from build123d import *

# Parameters (mm, degrees)
SKETCH1_R                = 10.5
BOSS_EXTRUDE1_DEPTH      = 2
SKETCH1_2_R              = 10.5
BOSS_EXTRUDE2_DEPTH      = 2
SKETCH2_R                = 12.5
SKETCH2_R_2              = 10.5
BOSS_EXTRUDE3_DEPTH      = 3.015
BOSS_EXTRUDE3_DEPTH_BACK = 3.015


with BuildPart() as part:
    # Sketch1 → Boss-Extrude1 (new body)
    with BuildSketch(Plane(origin=(0, 0, 0), x_dir=(1, 0, 0), z_dir=(0, 1, 0))):
        Circle(SKETCH1_R)
    extrude(amount=BOSS_EXTRUDE1_DEPTH)

    # Sketch1_2 → Boss-Extrude2 (add)
    with BuildSketch(Plane(origin=(0, 0, 0), x_dir=(1, 0, 0), z_dir=(0, 1, 0))):
        Circle(SKETCH1_2_R)
    extrude(amount=-BOSS_EXTRUDE2_DEPTH)

    # Sketch2 → Boss-Extrude3 (add, two sides)
    with BuildSketch(Plane(origin=(0, 0, 0), x_dir=(1, 0, 0), z_dir=(0, 1, 0))) as boss_extrude3_sk:
        Circle(SKETCH2_R)
        Circle(SKETCH2_R_2, mode=Mode.SUBTRACT)
    extrude(amount=BOSS_EXTRUDE3_DEPTH)
    extrude(boss_extrude3_sk.sketch, amount=-BOSS_EXTRUDE3_DEPTH_BACK)


solid = part.part
Part model, mm, in its own coordinate system. A direction names the side the tool comes from. Coordinates: 2 decimals unless noted, no trailing zeros. Order: outer loops, then holes, each group sorted by start corner. A loop starts at its lowest first (then second) coordinate and runs counter-clockwise, first axis right, second up. Notation, with made-up numbers: M 12.5,25 L 69.5,25 A16 cw 69.5,35 Z; hole C 84.5,-30.75 d5. An arc over 180 degrees is marked long. One line per question, with ' | ' between items.
Q1. Slice it at B-B (x = 0). Give the cut face in (y, z) (3 decimals), and give its area (3 significant figures).
A:
outline: M -3.015,-12.5 L 3.015,-12.5 L 3.015,-10.5 L 2,-10.5 L 2,10.5 L 3.015,10.5 L 3.015,12.5 L -3.015,12.5 L -3.015,10.5 L -2,10.5 L -2,-10.5 L -3.015,-10.5 Z | area: 108 mm^2
Q2. Pin check, flat tips, straight feed: P1, Ø2, axis at x = 1, z = -8.5, coming from the -Y side; P2, Ø1.5, axis at x = -6.5, y = 2.5, coming from the +Z side; P3, Ø1, axis at y = -0.5, z = 3.5, coming from the -X side; P4, Ø3, axis at x = 1, y = -2, coming from the +Z side. Stop position of each tip, or through.
A:
P1: stops at y = -2 | P2: stops at z = 11.1 | P3: stops at x = -12.13 | P4: stops at z = 12.5
Q3. Slice it at C-C (y = -1.25). Give the cut face in (x, z), and give its area (3 significant figures).
A:
outline: C 0,0 d25 | area: 491 mm^2
Q4. 3-axis set-ups, long thin cutter, end or side, ignore diameter. For faces 3 (the face through (0, -2, 0)), 4 (the face through (10, 2.5, -3.2)): which of +Z, -Z, +X, -X, +Y, -Y reach the whole face in a straight line?
A:
face 3: -Y | face 4: +Y
Q5. Two-plate mould, pull along X, no slides. Class faces 1 (the face through (11.923, 0.042, -3.755)), 2 (the face through (10, -2.5, -3.2)): +X half, -X half, draft (parallel to the pull), parting line (faces both ways), or undercut.
A:
face 1: parting line | face 2: undercut
Q6. Slice it at A-A (z = 0). Give the cut face in (x, y) (3 decimals), and give its area (3 significant figures).
A:
outline: M -12.5,-3.015 L -10.5,-3.015 L -10.5,-2 L 10.5,-2 L 10.5,-3.015 L 12.5,-3.015 L 12.5,3.015 L 10.5,3.015 L 10.5,2 L -10.5,2 L -10.5,3.015 L -12.5,3.015 Z | area: 108 mm^2
Q7. Drill centre lines: line 1 (Z direction, x = 0, y = 2.4); line 2 (Y direction, x = 6, z = 5). Where is each one in solid material? Low to high.
A:
line 1: z = -12.5 to -10.5, 10.5 to 12.5 | line 2: y = -2 to 2
